Check sheet for the modelled part. Datum: model origin and axes. Units: mm. Face numbers are marked on the shaded views. A direction names the side the tool comes from. Round coordinates to 2 decimals unless told otherwise and drop trailing zeros. Order: outer loops, then holes, each group sorted by start corner. A loop starts at its lowest first (then second) coordinate and runs counter-clockwise, first axis right, second up. Notation, with made-up numbers: (45, 33) -> (64, 33) arc R12 cw to (64, 50) -> close; hole circle Ø4 at (-39, 4.5). An arc over 180 degrees is marked (long way). Answer in a Markdown table with one row per item.
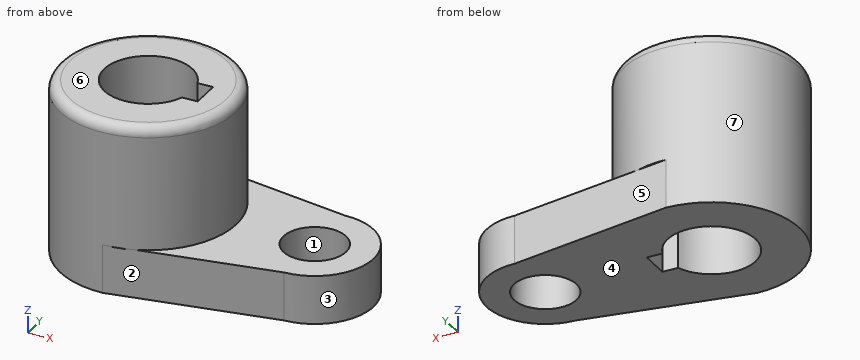
```python
from build123d import *

# Parameters (mm, degrees)
F0_R     = 10.16
F1_DEPTH = 15.7734
F2_R     = 28.575
F3_DEPTH = 40.2336
F4_R     = 3.302


with BuildPart() as f1:
    # F0 (on Top) → F1 (new body)
    with BuildSketch(Plane.XY):
        with BuildLine():
            Line((53.975, 19.05), (0, 28.575))
            ThreePointArc((0, 28.575), (-28.575, 0), (0, -28.575))
            Line((0, -28.575), (53.975, -19.05))
            ThreePointArc((53.975, -19.05), (73.025, 0), (53.975, 19.05))
        make_face()
        with BuildLine():
            ThreePointArc((13.447765, -4.826), (-14.2875, 0), (13.447765, 4.826))
            Line((13.447765, 4.826), (18.5293, 4.826))
            Line((18.5293, 4.826), (18.5293, -4.826))
            Line((18.5293, -4.826), (13.447765, -4.826))
        make_face(mode=Mode.SUBTRACT)
        with Locations((53.975, 0)):
            Circle(F0_R, mode=Mode.SUBTRACT)
    extrude(amount=F1_DEPTH)

    # F2 (on face) → F3 (join)
    with BuildSketch(Plane.XY.offset(15.7734)):
        Circle(F2_R)
        with BuildLine():
            ThreePointArc((13.447765, -4.826), (-14.2875, 0), (13.447765, 4.826))
            Line((13.447765, 4.826), (18.5293, 4.826))
            Line((18.5293, 4.826), (18.5293, -4.826))
            Line((18.5293, -4.826), (13.447765, -4.826))
        make_face(mode=Mode.SUBTRACT)
    extrude(amount=F3_DEPTH)

    # F4
    f4_edges = [f1.edges().sort_by_distance(p)[0] for p in [
        (-28.575, 0, 56.007),
    ]]
    fillet(f4_edges, radius=F4_R)


solid = f1.part
```
(1) Section check C-C on x = 50.5. Record the boundary of the cut face in (y, z), plus the area to 3 significant figures.
Solutions:
| item | result |
|---|---|
| outline | (-19.66, 0) -> (-9.55, 0) -> (-9.55, 15.77) -> (-19.66, 15.77) -> close; (9.55, 0) -> (19.66, 0) -> (19.66, 15.77) -> (9.55, 15.77) -> close |
| area | 319 mm^2 |
(2) Depth check by flat-ended pin: pin 1 Ø4 at (x, z) = (16, 32) entering from +Y; pin 2 Ø1.5 at (x, z) = (9.5, 16.5) entering from -Y; pin 3 Ø1.5 at (y, z) = (-18.5, 37) entering from +X. Enter the tip coordinate at first touch or a pass-through.
Solutions:
| item | result |
|---|---|
| pin 1 | y = 24.91 |
| pin 2 | y = -27.2 |
| pin 3 | x = 22.39 |
(3) Section check D-D on y = -8.5. Give the number of separate pieces and of enclosed holes in the cut face, plus the area to 3 significant figures.
Solutions:
| item | result |
|---|---|
| separate pieces | 3 |
| enclosed holes | 0 |
| area | 2,280 mm^2 |
(4) Section check A-A on y = 0. Record the boundary of the cut face in (x, z) (1 decimal).
Solutions:
| item | result |
|---|---|
| outline | (-28.6, 0) -> (-14.3, 0) -> (-14.3, 56) -> (-25.3, 56) arc R3.3 ccw to (-28.6, 52.7) -> close; (18.5, 0) -> (43.8, 0) -> (43.8, 15.8) -> (28.6, 15.8) -> (28.6, 52.7) arc R3.3 ccw to (25.3, 56) -> (18.5, 56) -> close; (64.1, 0) -> (73, 0) -> (73, 15.8) -> (64.1, 15.8) -> close |
(5) Scan lines: probe 1 along X at (y, z) = (0, 23) (1 decimal); probe 2 along Y at (x, z) = (0, 42.5) (1 decimal); probe 3 along Y at (x, z) = (54, 10.5). Record each from-to range of solid material in increasing order. Write a range as from..to.
Solutions:
| item | result |
|---|---|
| probe 1 | -28.6..-14.3, 18.5..28.6 |
| probe 2 | -28.6..-14.3, 14.3..28.6 |
| probe 3 | -19.05..-10.16, 10.16..19.05 |
(6) Tool access check on the marked faces 5, 6 and 7. Record the directions out of +Z, -Z, +X, -X, +Y, -Y that give a thin tool (end or side, any length) a straight path to the whole face; none if there is none.
Solutions:
| item | result |
|---|---|
| face 5 | -Z, +X, +Y |
| face 6 | +Z, +X, -X, +Y, -Y |
| face 7 | +Z |
(7) Draft check along Y on the marked faces 1, 2, 3 and 4. Enter one of: pulls with the +Y half, pulls with the -Y half, needs draft (parallel to the pull), parting line crosses it, or undercut.
Solutions:
| item | result |
|---|---|
| face 1 | undercut |
| face 2 | pulls with the -Y half |
| face 3 | parting line crosses it |
| face 4 | needs draft |
